Autodesk Inventor part; units mm, degrees
ref_plane "YZ Plane" through (0, 0, 0) normal (1, 0, 0) x (0, 1, 0)
ref_plane "XZ Plane" through (0, 0, 0) normal (0, 1, 0) x (-1, 0, 0)
ref_plane "XY Plane" through (0, 0, 0) normal (0, 0, 1) x (1, 0, 0)
sketch "Sketch1" plane through (0, 0, 0) normal (0, 0, 1) x (1, 0, 0)
  line L0 (0, 0) -> (228.6, 0)
  line L1 (228.6, 0) -> (354.3236, 125.7236)
  line L2 (354.3236, 125.7236) -> (352.0785, 127.9686)
  line L3 (352.0785, 127.9686) -> (227.2849, 3.175)
  line L4 (0, 0) -> (0, 3.175)
  line L5 (0, 3.175) -> (227.2849, 3.175)
  line L6 (0, 3.175) -> (0, 25.4)
  line L7 (0, 25.4) -> (217.2198, 25.4)
  line L8 (352.0785, 127.9686) -> (336.3631, 143.6841)
  line L9 (336.3631, 143.6841) -> (218.6865, 26.0075)
  line L10 (217.2198, 25.4) -> (226.2228, 3.665)
  line L11 (218.6865, 26.0075) -> (227.6894, 4.2725)
  arc A0 (226.2228, 3.665) -> (227.6894, 4.2725) centre (226.9561, 3.9688) ccw
  line L12 (217.2198, 25.4) -> (218.079, 25.4) construction
  line L13 (218.6865, 26.0075) -> (218.079, 25.4) construction
  dimension "d4" = 3.175
  dimension "d6" = 3.175
  dimension "d8" = 25.4
  dimension "d9" = 25.4
  dimension "d10" = 45
  dimension "d11" = 228.6
  dimension "d12" = 177.8
  dimension "d13" = 1.5875
extrude "Extrusion1" add sketch "Sketch1" along normal blind 3.175 contours L6 L7 L10 A0 L5 | A0 L3 L5 | L3 A0 L11 L9 L8
extrude "Extrusion2" add sketch "Sketch1" along normal blind 50.8 contours L4 L5 L3 L2 L1 L0
sketch "Sketch2" plane through (0, 0, 0) normal (0, -1, 0) x (1, 0, 0)
  line L0 (0, 0) -> (0, 50.8)
  line L1 (0, 0) -> (228.6, 0)
  line L2 (228.6, 0) -> (228.6, 50.8)
  circle A0 centre (25.4, 25.4) radius 14.2875
  circle A1 centre (203.2, 25.4) radius 14.2875
  dimension "d18" = 28.575
  dimension "d19" = 25.4
  dimension "d20" = 25.4
  dimension "d21" = 25.4
extrude "Extrusion3" cut sketch "Sketch2" against normal through all
equation "\"d4\" = d6"
properties part number "8 ball bottom 1 by 2 L"
Work out the finished part from the listing and answer in its coordinate system (mm). A direction names the side the tool comes from. Give positions to 0.01 mm unless a question says otherwise; leave off trailing zeros. Loops run counter-clockwise (first coordinate to the right, second up) from the corner with the lowest first, then second, coordinate; pieces in that order, holes last. Notation, with made-up numbers: (69.5, 58) -> (113.5, 58) arc R11 cw to (113.5, 76) -> close; hole circle Ø5 at (63, -12). An arc over 180 degrees is marked (long way). Write item = value, one per line. Start each with the question number.
(1) The mould has two halves that part along Y. Classify faces 4 (the flat face through (221.66, 14.68, 1.57)), 5 (the flat face through (112, 14, 3.175)), 6 (the flat face through (113, 0, 25)): +Y half, -Y half, draft (parallel to the pull), parting line (faces both ways), or undercut.
(2) Find section D-D on y = 39.5. Give the vertices of the cut face in (x, z) (3 decimals).
(3) Which of the six approach directions +Z, -Z, +X, -X, +Y, -Y give full straight-line access (tool end or side, diameter ignored) to faces 1 (the flat face through (285, 74, 3.175)), 2 (the cylindrical face through (11.126, 1.565, 26.028)), 3 (the flat face through (223.125, 15.292, 1.565))?
(4) Find section A-A on z = 25.4. Give the vertices of the cut face in (x, y) (1 decimal), and give its area (3 significant figures).
(5) Find section C-C on z = 47. Give the vertices of the cut face in (x, y) (1 decimal).
(6) Find the intervals of material crossed by probe 1 along Z at (x, y) = (203, 2); probe 2 along X at (y, z) = (1, 25); probe 3 along Y at (x, z) = (209, 38.5) (3 decimals), in increasing order. Write a range as from..to.
(7) Given pin 1 Ø8 at (x, z) = (310, 8) entering from -Y; pin 2 Ø10 at (x, z) = (284.5, 15.5) entering from +Y; pin 3 Ø24 at (x, z) = (117, 28) entering from +Y (3 decimals), each flat-ended and moving along its own axis, determine where each tip first touches the part or whether it passes through.
(8) Find section B-B on x = 25.4. Give the vertices of the cut face in (y, z) (1 decimal).
From the geometry:
q1.face_4 = undercut
q1.face_5 = draft
q1.face_6 = -Y half
q2.outline = (232.179, 0) -> (268.1, 0) -> (268.1, 50.8) -> (263.61, 50.8) -> (263.61, 3.175) -> (232.179, 3.175) -> close
q3.face_1 = +Z, -X, +Y
q3.face_2 = +Y, -Y
q3.face_3 = +Z, -Z
q4.outline = (0, 0) -> (11.1, 0) -> (11.1, 3.2) -> (0, 3.2) -> close; (39.7, 0) -> (188.9, 0) -> (188.9, 3.2) -> (39.7, 3.2) -> close; (217.5, 0) -> (228.6, 0) -> (354.3, 125.7) -> (352.1, 128) -> (227.3, 3.2) -> (217.5, 3.2) -> close
q4.area = 1,100 mm^2
q5.outline = (0, 0) -> (228.6, 0) -> (354.3, 125.7) -> (352.1, 128) -> (227.3, 3.2) -> (0, 3.2) -> close
q6.probe_1 = 0..11.11, 39.69..50.8
q6.probe_2 = 0..11.12, 39.68..188.92, 217.48..229.6
q6.probe_3 = 0..3.175
q7.pin_1 = 77.4
q7.pin_2 = 65.39
q7.pin_3 = 3.175
q8.outline = (0, 0) -> (25.4, 0) -> (25.4, 3.2) -> (3.2, 3.2) -> (3.2, 11.1) -> (0, 11.1) -> close; (0, 39.7) -> (3.2, 39.7) -> (3.2, 50.8) -> (0, 50.8) -> close
